Check sheet for the modelled part. Datum: model origin and axes. Units: mm. A direction names the side the tool comes from. Coordinates: 2 decimals unless noted, no trailing zeros. Order: outer loops, then holes, each group sorted by start corner. A loop starts at its lowest first (then second) coordinate and runs counter-clockwise, first axis right, second up. Notation, with made-up numbers: (-3.5, -39) -> (46.5, -39) arc R15 cw to (46.5, -32) -> close; hole circle Ø10 at (-12, 40.25). An arc over 180 degrees is marked (long way). Put each result on its own line as item: value. Start each with the question number.
```python
from build123d import *

# Parameters (mm, degrees)
SKETCH1_W           = 6
SKETCH1_H           = 6
BOSS_EXTRUDE1_DEPTH = 5
CUT_EXTRUDE1_DEPTH  = 10
CUT_EXTRUDE2_DEPTH  = 3


with BuildPart() as part:
    # Sketch1 → Boss-Extrude1 (new body)
    with BuildSketch(Plane(origin=(0, 0, 0), x_dir=(1, 0, 0), z_dir=(0, 1, 0))):
        Rectangle(SKETCH1_W, SKETCH1_H)
    extrude(amount=BOSS_EXTRUDE1_DEPTH)

    # Sketch2 → Cut-Extrude1 (cut)
    with BuildSketch(Plane.ZY.offset(3)):
        Polygon((3, 5), (-3, 5), (0, 2.5), (3, 2.5), align=None)
    extrude(amount=-CUT_EXTRUDE1_DEPTH, mode=Mode.SUBTRACT)

    # Sketch3 → Cut-Extrude2 (cut)
    with BuildSketch(Plane(origin=(3, 0, 0), x_dir=(0, 0, -1), z_dir=(1, 0, 0))):
        Polygon((-3, 0), (0, 2.5), (-3, 2.5), align=None)
    extrude(amount=-CUT_EXTRUDE2_DEPTH, mode=Mode.SUBTRACT)


solid = part.part
```
1) Sectioned sample at C-C (z = -0.3). Record the boundary of the cut face in (x, y).
2) Scan lines: line 1 along Y through (x, z) = (2.45, 0); line 2 along X through (y, z) = (2.2, 1.2); line 3 along Z through (x, y) = (1.3, 1.9). Record each from-to range of solid material in increasing order. Write a range as [from, to].
3) Gauge pin test, flat ends, axial feed: pin 1 (3.5 mm diameter, centred on x = -2, z = 1.5, fed in from +Y); pin 2 (2 mm diameter, centred on y = 4, z = 2, fed in from +X). Record the tip position at first contact, or that the pin passes through.
4) Access from +Z, -Z, +X, -X, +Y, -Y to the whole of each face (thin tool, end or side, straight path). Record for faces 1 (the flat face through (3, 1, -1)), 2 (the flat face through (0, 2, 2)), 3 (the flat face through (-2, 2.5, 1)).
5) Sectioned sample at A-A (y = 1.85). Record the boundary of the cut face in (x, z).
6) Sectioned sample at D-D (y = 4.45). Record the boundary of the cut face in (x, z), plus the area to 3 significant figures.
7) Sectioned sample at B-B (x = -1.45). Record the boundary of the cut face in (y, z).
Entries:
1. outline: (-3, 0) -> (3, 0) -> (3, 2.75) -> (-3, 2.75) -> close
2. line 1: y = [0, 2.5]
2. line 2: x = [-3, 0]
2. line 3: z = [-3, 0.72]
3. pin 1: stops at y = 2.71
3. pin 2: passes through
4. face 1: +Z, -Z, +X, +Y, -Y
4. face 2: +Z, +X, +Y
4. face 3: +Z, +X, -X, +Y
5. outline: (-3, -3) -> (3, -3) -> (3, 0.78) -> (0, 0.78) -> (0, 3) -> (-3, 3) -> close
6. outline: (-3, -3) -> (3, -3) -> (3, -2.34) -> (-3, -2.34) -> close
6. area: 3.96 mm2
7. outline: (0, -3) -> (5, -3) -> (2.5, 0) -> (2.5, 3) -> (0, 3) -> close
